from build123d import *

# Parameters (mm, degrees)
F0_R     = 45
F1_DEPTH = 3


with BuildPart() as f1:
    # F0 (on Top) → F1 (new body)
    with BuildSketch(Plane.XY):
        with BuildLine():
            Line((49.963624, 2), (54.963624, 2))
            ThreePointArc((54.963624, 2), (50.813374, 21.047589), (40.279365, 37.450938))
            Line((40.279365, 37.450938), (36.743831, 33.915404))
            Line((36.743831, 33.915404), (33.915404, 36.743831))
            Line((33.915404, 36.743831), (37.450938, 40.279365))
            ThreePointArc((37.450938, 40.279365), (21.047589, 50.813374), (2, 54.963624))
            Line((2, 54.963624), (2, 49.963624))
            Line((2, 49.963624), (-2, 49.963624))
            Line((-2, 49.963624), (-2, 54.963624))
            ThreePointArc((-2, 54.963624), (-21.047589, 50.813374), (-37.450938, 40.279365))
            Line((-37.450938, 40.279365), (-33.915404, 36.743831))
            Line((-33.915404, 36.743831), (-36.743831, 33.915404))
            Line((-36.743831, 33.915404), (-40.279365, 37.450938))
            ThreePointArc((-40.279365, 37.450938), (-50.813374, 21.047589), (-54.963624, 2))
            Line((-54.963624, 2), (-49.963624, 2))
            Line((-49.963624, 2), (-49.963624, -2))
            Line((-49.963624, -2), (-54.963624, -2))
            ThreePointArc((-54.963624, -2), (-50.813374, -21.047589), (-40.279365, -37.450938))
            Line((-40.279365, -37.450938), (-36.743831, -33.915404))
            Line((-36.743831, -33.915404), (-33.915404, -36.743831))
            Line((-33.915404, -36.743831), (-37.450938, -40.279365))
            ThreePointArc((-37.450938, -40.279365), (-21.047589, -50.813374), (-2, -54.963624))
            Line((-2, -54.963624), (-2, -49.963624))
            Line((-2, -49.963624), (0, -49.963624))
            Line((0, -49.963624), (2, -49.963624))
            Line((2, -49.963624), (2, -54.963624))
            ThreePointArc((2, -54.963624), (21.047589, -50.813374), (37.450938, -40.279365))
            Line((37.450938, -40.279365), (33.915404, -36.743831))
            Line((33.915404, -36.743831), (36.743831, -33.915404))
            Line((36.743831, -33.915404), (40.279365, -37.450938))
            ThreePointArc((40.279365, -37.450938), (50.813374, -21.047589), (54.963624, -2))
            Line((54.963624, -2), (49.963624, -2))
            Line((49.963624, -2), (49.963624, 2))
        make_face()
        Circle(F0_R, mode=Mode.SUBTRACT)
    extrude(amount=F1_DEPTH)


solid = f1.part
Source: CAD feature listing. Evaluate the final solid. Frame: model axes, mm. A direction names the side the tool comes from. Give positions to 0.01 mm unless a question says otherwise; leave off trailing zeros. Loops run counter-clockwise (first coordinate to the right, second up) from the corner with the lowest first, then second, coordinate; pieces in that order, holes last. Notation, with made-up numbers: (-21.5, 7) -> (1.5, 7) arc R18 ccw to (1.5, 21) -> close; hole circle Ø5 at (-34, 85.5). An arc over 180 degrees is marked (long way). Use a Markdown table: item, result. Add a question column.
1) Section query A-A, the plane y = 0. Return the cut outline in (x, z).
2) Pull-direction query (Y, two-part tool) for faces 4 (the face through (35.31, -35.35, 1.48)), 5 (the face through (-2, 52, 1)), 6 (the face through (21.3, 50.71, 1.48)); classes: +Y half, -Y half, draft (parallel to the pull), parting line (faces both ways), or undercut.
3) First-contact query: pin 1 (1.5 mm diameter, centred on y = 0.5, z = 1.5, fed in from -X); pin 2 (0.9 mm diameter, centred on x = 0.5, z = 1.5, fed in from -Y); pin 3 (1.5 mm diameter, centred on y = 51.5, z = 1.5, fed in from -X). Flat tips, straight axial feed; report the tip coordinate or a pass-through.
4) Reachability of faces 1 (the face through (0, 49.964, 1)), 2 (the face through (-35.35, -35.31, 1.48)), 3 (the face through (52, 2, 1)) from +Z, -Z, +X, -X, +Y, -Y: full face, straight path, thin tool, end or side. Return the list, or none.
5) Line query: line 1 along Y through (x, z) = (0, 1.75); line 2 along X through (y, z) = (34, 0.4); line 3 along Y through (x, z) = (-28.5, 1.2). Output: solid intervals per line, ascending. Write a range as [from, to].
Numbers:
| question | item | result |
|---|---|---|
| 1 | outline | (-49.96, 0) -> (-45, 0) -> (-45, 3) -> (-49.96, 3) -> close; (45, 0) -> (49.96, 0) -> (49.96, 3) -> (45, 3) -> close |
| 2 | face 4 | undercut |
| 2 | face 5 | draft |
| 2 | face 6 | +Y half |
| 3 | pin 1 | stops at x = -49.96 |
| 3 | pin 2 | stops at y = -49.96 |
| 3 | pin 3 | stops at x = -21.2 |
| 4 | face 1 | +Z, -Z, +Y |
| 4 | face 2 | +Z, -Z |
| 4 | face 3 | +Z, -Z, +X |
| 5 | line 1 | y = [-49.96, -45], [45, 49.96] |
| 5 | line 2 | x = [-43.23, -36.83], [-36.66, -29.48], [29.48, 36.66], [36.83, 43.23] |
| 5 | line 3 | y = [-47.04, -34.82], [34.82, 47.04] |
